Could you check a few things on this model? Use its own coordinates, in mm. A direction names the side the tool comes from. Round coordinates to 2 decimals unless told otherwise and drop trailing zeros. Loops run counter-clockwise (first coordinate to the right, second up) from the corner with the lowest first, then second, coordinate; pieces in that order, holes last. Notation, with made-up numbers: M 30,28 L 73,28 A27 ccw 73,49 Z; hole C -17,81.5 d11. An arc over 180 degrees is marked long. Answer in a Markdown table with one row per item.
```python
from build123d import *

# Parameters (mm, degrees)
PAD_DEPTH       = 4
POCKET003_DEPTH = 3
POCKET004_DEPTH = 32.001
SKETCH012_W     = 3.1
SKETCH012_H     = 2
POCKET006_DEPTH = 1
SKETCH013_W     = 2.1
SKETCH013_H     = 2
POCKET007_DEPTH = 1
SKETCH014_W     = 2.1
SKETCH014_H     = 2
POCKET008_DEPTH = 1
SKETCH016_W     = 1
SKETCH016_H     = 1
POCKET009_DEPTH = 2
SKETCH018_W     = 1
SKETCH018_H     = 1
POCKET010_DEPTH = 1
SKETCH021_R     = 12
POCKET011_DEPTH = 0.2
SKETCH024_W     = 1.35
SKETCH024_H     = 1.1
SKETCH024_W_2   = 1.1
SKETCH024_H_2   = 1.35
POCKET012_DEPTH = 1.2
BOX009_W        = 1
BOX009_H        = 8
BOX009_DEPTH    = 3
BOX010_W        = 6
BOX010_H        = 1
BOX010_DEPTH    = 3
BOX008_W        = 6
BOX008_H        = 1
BOX008_DEPTH    = 3
PAD007_DEPTH    = 1
FILLET_R        = 0.3
FILLET009_R     = 0.3


with BuildPart() as pocket012:
    # Sketch001 → Pad (new body)
    with BuildSketch(Plane(origin=(13.75, 21, 0), x_dir=(1, 0, 0), z_dir=(0, 0, 1))):
        with BuildLine():
            ThreePointArc((16, 22), (0, 24.8188), (-16, 22))
            Line((-16, 22), (-16, -22))
            ThreePointArc((-16, -22), (0, -24.8188), (16, -22))
            Line((16, -22), (16, 22))
        make_face()
    extrude(amount=PAD_DEPTH)

    # Sketch005 → Pocket003 (cut)
    with BuildSketch(Plane(origin=(13.75, 21, 0), x_dir=(1, 0, 0), z_dir=(0, 0, -1))):
        with BuildLine():
            Line((14, 21.25), (14, -21.25))
            Line((8.799858, -21.25), (14, -21.25))
            ThreePointArc((-8.799858, -21.25), (0, -23), (8.799858, -21.25))
            Line((-8.799858, -21.25), (-14, -21.25))
            Line((-14, -21.25), (-14, 21.25))
            Line((-14, 21.25), (-8.799858, 21.25))
            ThreePointArc((-3, 22.803509), (-5.950841, 22.216829), (-8.799858, 21.25))
            Line((3, 22.803509), (-3, 22.803509))
            ThreePointArc((8.799858, 21.25), (5.950841, 22.216829), (3, 22.803509))
            Line((8.799858, 21.25), (14, 21.25))
        make_face()
    extrude(amount=-POCKET003_DEPTH, mode=Mode.SUBTRACT)

    # Sketch007 → Pocket004 (cut, through all)
    with BuildSketch(Plane(origin=(-2.25, 21, 0), x_dir=(0, -1, 0), z_dir=(-1, 0, 0))):
        with BuildLine():
            ThreePointArc((-1.05, 2.6), (-1.85, 1.8), (-1.05, 1))
            Line((-1.05, 1), (3.85, 1))
            ThreePointArc((3.85, 1), (4.65, 1.8), (3.85, 2.6))
            Line((-1.05, 2.6), (3.85, 2.6))
        make_face()
    extrude(amount=-POCKET004_DEPTH, mode=Mode.SUBTRACT)

    # Sketch012 → Pocket006 (cut)
    with BuildSketch(Plane(origin=(13.75, -1.803509, 0), x_dir=(-1, 0, 0), z_dir=(0, 1, 0))):
        with Locations((0, 2)):
            Rectangle(SKETCH012_W, SKETCH012_H)
    extrude(amount=-POCKET006_DEPTH, mode=Mode.SUBTRACT)

    # Sketch013 → Pocket007 (cut)
    with BuildSketch(Plane(origin=(-0.25, 21, 0), x_dir=(0, 1, 0), z_dir=(1, 0, 0))):
        with Locations((20, 2)):
            Rectangle(SKETCH013_W, SKETCH013_H)
    extrude(amount=-POCKET007_DEPTH, mode=Mode.SUBTRACT)

    # Sketch014 → Pocket008 (cut)
    with BuildSketch(Plane(origin=(27.75, 21, 0), x_dir=(0, -1, 0), z_dir=(-1, 0, 0))):
        with Locations((-20, 2)):
            Rectangle(SKETCH014_W, SKETCH014_H)
    extrude(amount=-POCKET008_DEPTH, mode=Mode.SUBTRACT)

    # Sketch016 → Pocket009 (cut)
    with BuildSketch(Plane(origin=(-2.25, 21, 0), x_dir=(0, -1, 0), z_dir=(-1, 0, 0))):
        with Locations((13, 2)):
            Rectangle(SKETCH016_W, SKETCH016_H)
        with Locations((15, 2)):
            Rectangle(SKETCH016_W, SKETCH016_H)
        with Locations((17, 2)):
            Rectangle(SKETCH016_W, SKETCH016_H)
    extrude(amount=-POCKET009_DEPTH, mode=Mode.SUBTRACT)

    # Sketch018 → Pocket010 (cut)
    with BuildSketch(Plane(origin=(13.75, 21, 4), x_dir=(1, 0, 0), z_dir=(0, 0, 1))):
        with Locations((-10.5, -13)):
            Rectangle(SKETCH018_W, SKETCH018_H)
        with Locations((-10.5, -15)):
            Rectangle(SKETCH018_W, SKETCH018_H)
        with Locations((-10.5, -17)):
            Rectangle(SKETCH018_W, SKETCH018_H)
        with Locations((-12.5, -14)):
            Rectangle(SKETCH018_W, SKETCH018_H)
        with Locations((-12.5, -16)):
            Rectangle(SKETCH018_W, SKETCH018_H)
    extrude(amount=-POCKET010_DEPTH, mode=Mode.SUBTRACT)

    # Sketch021 → Pocket011 (cut)
    with BuildSketch(Plane(origin=(13.75, 21, 3), x_dir=(1, 0, 0), z_dir=(0, 0, -1))):
        with Locations((0, -10.5)):
            Circle(SKETCH021_R)
    extrude(amount=-POCKET011_DEPTH, mode=Mode.SUBTRACT)

    # Sketch024 → Pocket012 (cut)
    with BuildSketch(Plane(origin=(13.75, 21, 0), x_dir=(1, 0, 0), z_dir=(0, 0, -1))):
        with Locations((-9.55, 21.8)):
            Rectangle(SKETCH024_W, SKETCH024_H)
        with Locations((9.45, 21.8)):
            Rectangle(SKETCH024_W, SKETCH024_H)
        with Locations((-14.55, -16.4)):
            Rectangle(SKETCH024_W_2, SKETCH024_H_2)
        with Locations((14.55, -16.4)):
            Rectangle(SKETCH024_W_2, SKETCH024_H_2)
    extrude(amount=-POCKET012_DEPTH, mode=Mode.SUBTRACT)


with BuildPart() as box009:
    # Box009 → Box009 (new body)
    with BuildSketch(Plane(origin=(5.5, 2, 0), x_dir=(1, 0, 0), z_dir=(0, 0, 1))):
        with Locations((0.5, 4)):
            Rectangle(BOX009_W, BOX009_H)
    extrude(amount=BOX009_DEPTH)


with BuildPart() as box010:
    # Box010 → Box010 (new body)
    with BuildSketch(Plane(origin=(-0.5, 2, 0), x_dir=(1, 0, 0), z_dir=(0, 0, 1))):
        with Locations((3, 0.5)):
            Rectangle(BOX010_W, BOX010_H)
    extrude(amount=BOX010_DEPTH)


with BuildPart() as fusion013:
    # Box008 → Box008 (new body)
    with BuildSketch(Plane(origin=(-0.5, 9, 0), x_dir=(1, 0, 0), z_dir=(0, 0, 1))):
        with Locations((3, 0.5)):
            Rectangle(BOX008_W, BOX008_H)
    extrude(amount=BOX008_DEPTH)

    # Fusion012: union Box009, Box010
    add(box009.part)
    add(box010.part)

    # Fusion013: union Pocket012
    add(pocket012.part)


with BuildPart() as fillet009:
    # Sketch025 → Pad007 (new body)
    with BuildSketch(Plane(origin=(13.5, 1, 0), x_dir=(1, 0, 0), z_dir=(0, 0, 1))):
        with BuildLine():
            ThreePointArc((5, 48), (0, 48.266714), (-5, 48))
            Line((-5, 48), (-5, 44))
            Line((-5, 44), (-3.5, 44))
            Line((-3.5, 47), (-3.5, 44))
            ThreePointArc((3.5, 47), (0, 47.130139), (-3.5, 47))
            Line((3.5, 44), (3.5, 47))
            Line((5, 44), (3.5, 44))
            Line((5, 48), (5, 44))
        make_face()
    extrude(amount=PAD007_DEPTH)

    # Fusion014: union Fusion013
    add(fusion013.part)

    # Fillet
    fillet_edges = [fillet009.edges().sort_by_distance(p)[0] for p in [
        (13.75, 45.8188, 4),
        (29.75, 21, 4),
        (29.75, 43, 2),
        (18.5, 47.28861, 1),
        (13.5, 49.266714, 1),
        (8.5, 47.261758, 1),
        (10, 46.834189, 1),
        (13.5, 48.130139, 1),
        (17, 46.852931, 1),
        (-2.25, 43, 2),
        (-2.25, 21, 4),
        (-2.25, -1, 2),
        (13.75, -3.8188, 4),
        (29.75, -1, 2),
    ]]
    fillet(fillet_edges, radius=FILLET_R)

    # Fillet009
    fillet009_edges = [fillet009.edges().sort_by_distance(p)[0] for p in [
        (8.5, 49, 0.35),
        (18.5, 49, 0.35),
    ]]
    fillet(fillet009_edges, radius=FILLET009_R)


solid = fillet009.part
```
1) Will these pins go through, and if not, where does the flat tip stop? P1, Ø10, axis at x = 7, y = 15.5, coming from the -Z side; P2, Ø0.9, axis at x = 26, z = 1.5, coming from the -Y side; P3, Ø0.6, axis at x = -0.5, y = 37.5, coming from the -Z side.
Computed:
| item | result |
|---|---|
| P1 | stops at z = 3 |
| P2 | stops at y = -2.31 |
| P3 | stops at z = 1.2 |
2) I want a section at A-A, the plane y = 7. Please give me the cut outline in (x, z).
Computed:
| item | result |
|---|---|
| outline | M -2.25,0 L -0.25,0 L -0.25,3 L 0.75,3 L 0.75,4 L -1.95,4 A0.3 ccw -2.25,3.7 Z; M 1.75,3 L 5.5,3 L 5.5,0 L 6.5,0 L 6.5,3 L 27.75,3 L 27.75,0 L 29.75,0 L 29.75,3.7 A0.3 ccw 29.45,4 L 1.75,4 Z |
3) If we mould it in two halves opening along Z, with no side actions, what happens to faces 6 (the face through (13.1, 48.7, 1)), 7 (the face through (3.2, 6.5, 3.5)), 8 (the face through (14, -2, 1)), 9 (the face through (15.3, -2, 2))? For each: released by +Z, released by -Z, zero draft, split by the parting line, or undercut.
Computed:
| item | result |
|---|---|
| face 6 | released by +Z |
| face 7 | zero draft |
| face 8 | undercut |
| face 9 | undercut |
4) I need wall thicknesses on line 1 (X direction, y = 28, z = 1.9); line 2 (Y direction, x = 4, z = 1.15). Which ranges of each line are inside material? Lowest first, please.
Computed:
| item | result |
|---|---|
| line 1 | x = -2.25 to -0.25, 27.75 to 29.75 |
| line 2 | y = -2.79 to -1.35, 2 to 3, 9 to 10, 42.25 to 44.79 |
5) I want a section at B-B, the plane y = 18.5. Please give me the cut outline in (x, z), plus the area to 3 significant figures.
Computed:
| item | result |
|---|---|
| outline | M -2.25,0 L -0.25,0 L -0.25,1 L -2.25,1 Z; M -2.25,2.6 L -0.25,2.6 L -0.25,3 L 27.75,3 L 27.75,2.6 L 29.75,2.6 L 29.75,3.7 A0.3 ccw 29.45,4 L -1.95,4 A0.3 ccw -2.25,3.7 Z; M 27.75,0 L 29.75,0 L 29.75,1 L 27.75,1 Z |
| area | 37.6 mm² |
6) Which directions (+Z, -Z, +X, -X, +Y, -Y) give clear straight access to the entire face, cutting with the end or side of a thin tool? Please do faces 1 (the face through (-1, 6, 2.5)), 2 (the face through (14, 21, 4)), 3 (the face through (2.75, 8, 3.5)), 4 (the face through (-1, 39.95, 2)), 5 (the face through (23.875, -1, 1)).
Computed:
| item | result |
|---|---|
| face 1 | -X |
| face 2 | +Z, +X, -X, +Y, -Y |
| face 3 | +Z, -Z |
| face 4 | none |
| face 5 | -Z |
7) I want a section at C-C, the plane y = 31.5. Please give me the cut outline in (x, z).
Computed:
| item | result |
|---|---|
| outline | M -2.25,0 L -0.25,0 L -0.25,3 L 1.75,3 L 1.75,3.2 L 25.75,3.2 L 25.75,3 L 27.75,3 L 27.75,0 L 29.75,0 L 29.75,3.7 A0.3 ccw 29.45,4 L -1.95,4 A0.3 ccw -2.25,3.7 Z |
